```python
from build123d import *

# Parameters (mm, degrees)
F0_W     = 8.3
F0_H     = 5
F1_DEPTH = 17.9
F2_W     = 7.9
F2_H     = 3.622741
F2_H_2   = 3.610624
F2_H_3   = 3.642021
F2_H_4   = 3.108276
F2_H_5   = 2.429072
F3_DEPTH = 25
F4_W     = 4.4
F4_H     = 3.622741
F4_H_2   = 3.610624
F4_H_3   = 3.642021
F4_H_4   = 3.108276
F4_H_5   = 2.429072
F5_DEPTH = 25


with BuildPart() as f1:
    # F0 (on Top) → F1 (new body)
    with BuildSketch(Plane.XY):
        with Locations((4.15, -2.5)):
            Rectangle(F0_W, F0_H)
    extrude(amount=F1_DEPTH)

    # F2 (on face) → F3 (cut)
    with BuildSketch(Plane(origin=(0, 0, 0), x_dir=(-1, 0, 0), z_dir=(0, 1, 0))):
        with Locations((-4.15, 15.88863)):
            Rectangle(F2_W, F2_H)
        with Locations((-4.15, 11.86379)):
            Rectangle(F2_W, F2_H_2)
        with Locations((-4.15, 7.9235)):
            Rectangle(F2_W, F2_H_3)
        with Locations((-4.15, 4.234384)):
            Rectangle(F2_W, F2_H_4)
        with Locations((-4.15, 1.214536)):
            Rectangle(F2_W, F2_H_5)
    extrude(amount=-F3_DEPTH, mode=Mode.SUBTRACT)

    # F4 (on Right) → F5 (cut)
    with BuildSketch(Plane.YZ):
        with Locations((-2.5, 15.88863)):
            Rectangle(F4_W, F4_H)
        with Locations((-2.5, 11.86379)):
            Rectangle(F4_W, F4_H_2)
        with Locations((-2.5, 7.9235)):
            Rectangle(F4_W, F4_H_3)
        with Locations((-2.5, 4.234384)):
            Rectangle(F4_W, F4_H_4)
        with Locations((-2.5, 1.214536)):
            Rectangle(F4_W, F4_H_5)
    extrude(amount=F5_DEPTH, mode=Mode.SUBTRACT)


solid = f1.part
```
CAD build for the part. Positions are in the model's coordinates, mm. Coordinates: 2 decimals unless noted, no trailing zeros. Write each loop counter-clockwise with the first axis right and the second up, starting at its lowest first coordinate (ties: lowest second). Pieces come first, ordered by that corner, then holes. Notation, with made-up numbers: (23.25, 0.25) -> (39.25, 0.25) arc R19 cw to (39.25, 8.25) -> close; hole circle Ø5 at (63.5, 37). An arc over 180 degrees is marked (long way). Return JSON: item names as keys, results as strings. Group by question number.
Q1. Cut at A-A, the plane z = 12.75. Give the cut face in (x, y), then the cut area to 3 significant figures.
Q2. Pull direction Z, two halves, no side cores. Call faces 1 (the face through (4, -3, 14.077)), 2 (the face through (4, -2, 17.9)): released by +Z, released by -Z, zero draft, split by the parting line, or undercut.
Q3. Flat gauge pin, fed straight in: pin 1 (1.5 mm diameter, centred on x = 3, y = -3, fed in from -Z). Where does the tip first touch, or does it go through?
Q4. Cut at C-C, the plane x = 3.25. Give the cut face in (y, z).
Q5. Drill centre lines: line 1 (Z direction, x = 2.75, y = -2.15); line 2 (X direction, y = -4.8, z = 2). Where is each one in solid material? Low to high.
Q6. Cut at B-B, the plane y = -1.6. Give the cut face in (x, z).
Returned:
{
 "1": {"outline": "(0, -5) -> (0.2, -5) -> (0.2, -4.7) -> (0, -4.7) -> close; (0, -0.3) -> (0.2, -0.3) -> (0.2, 0) -> (0, 0) -> close; (8.1, -5) -> (8.3, -5) -> (8.3, -4.7) -> (8.1, -4.7) -> close; (8.1, -0.3) -> (8.3, -0.3) -> (8.3, 0) -> (8.1, 0) -> close", "area": "0.240 mm2"},
 "2": {"face 1": "undercut", "face 2": "released by +Z"},
 "3": {"pin 1": "stops at z = 2.43"},
 "4": {"outline": "(-5, 2.43) -> (0, 2.43) -> (0, 2.68) -> (-5, 2.68) -> close; (-5, 5.79) -> (0, 5.79) -> (0, 6.1) -> (-5, 6.1) -> close; (-5, 9.74) -> (0, 9.74) -> (0, 10.06) -> (-5, 10.06) -> close; (-5, 13.67) -> (0, 13.67) -> (0, 14.08) -> (-5, 14.08) -> close; (-5, 17.7) -> (0, 17.7) -> (0, 17.9) -> (-5, 17.9) -> close"},
 "5": {"line 1": "z = 2.43 to 2.68, 5.79 to 6.1, 9.74 to 10.06, 13.67 to 14.08, 17.7 to 17.9", "line 2": "x = 0 to 0.2, 8.1 to 8.3"},
 "6": {"outline": "(0, 2.43) -> (8.3, 2.43) -> (8.3, 2.68) -> (0, 2.68) -> close; (0, 5.79) -> (8.3, 5.79) -> (8.3, 6.1) -> (0, 6.1) -> close; (0, 9.74) -> (8.3, 9.74) -> (8.3, 10.06) -> (0, 10.06) -> close; (0, 13.67) -> (8.3, 13.67) -> (8.3, 14.08) -> (0, 14.08) -> close; (0, 17.7) -> (8.3, 17.7) -> (8.3, 17.9) -> (0, 17.9) -> close"}
}
